Source: CAD feature listing. Evaluate the final solid. Frame: model axes, mm. A direction names the side the tool comes from. Round coordinates to 2 decimals unless told otherwise and drop trailing zeros. Loops run counter-clockwise (first coordinate to the right, second up) from the corner with the lowest first, then second, coordinate; pieces in that order, holes last. Notation, with made-up numbers: (21.25, 25) - (75.25, 25) arc R23 ccw to (75.25, 43) - close; hole circle Ø9 at (-23, 62.5). An arc over 180 degrees is marked (long way). One line per question, with ' | ' between items.
from build123d import *

# Parameters (mm, degrees)
SKETCH2_R           = 13.5
BOSS_EXTRUDE1_DEPTH = 8
SKETCH3_W           = 30
SKETCH3_H           = 34.126910457
BOSS_EXTRUDE2_DEPTH = 8
FILLET1_R           = 1


with BuildPart() as part:
    # Sketch2 → Boss-Extrude1 (new body)
    with BuildSketch(Plane.XY):
        with BuildLine():
            Line((22.912878475, 16.112283523), (-0.087121525, 16.112283523))
            Line((-0.087121525, 16.112283523), (-0.087121525, -17.887716477))
            Line((-0.087121525, -17.887716477), (22.912878475, -17.887716477))
            ThreePointArc((22.912878475, -17.887716477), (39.912878475, -0.887716477), (22.912878475, 16.112283523))
        make_face()
        with Locations((22.912878475, -0.887716477)):
            Circle(SKETCH2_R, mode=Mode.SUBTRACT)
    extrude(amount=BOSS_EXTRUDE1_DEPTH)

    # Sketch3 → Boss-Extrude2 (add)
    with BuildSketch(Plane.ZY.offset(0.087121525)):
        with Locations((4, -0.824261249)):
            Rectangle(SKETCH3_W, SKETCH3_H)
    extrude(amount=-BOSS_EXTRUDE2_DEPTH)

    # Fillet1
    fillet1_edges = [part.edges().sort_by_distance(p)[0] for p in [
        (7.912878475, -0.887716477, 8),
        (7.912878475, -0.887716477, 0),
    ]]
    fillet(fillet1_edges, radius=FILLET1_R)


solid = part.part
1. Section query B-B, the plane z = 6.5. Return loops of the section in (x, y), plus the area to 3 significant figures.
Worked out:
outline: (-0.09, -17.89) - (22.91, -17.89) arc R17 ccw to (22.91, 16.11) - (7.91, 16.11) - (7.91, 16.24) - (-0.09, 16.24) - close; hole circle Ø27 at (22.91, -0.89) | area: 664 mm2
2. Contact query for flat-ended pins moving along their axis: P1, Ø5, axis at x = 33.5, y = 10.5, coming from the +Z side; P2, Ø5, axis at x = 19.5, z = 2.5, coming from the +Y side; P3, Ø8, axis at y = -11.5, z = -0.5, coming from the +X side; P4, Ø6, axis at x = 19, z = -5.5, coming from the -Y side. Output: stop coordinate, or through.
Worked out:
P1: stops at z = 8 | P2: stops at y = 16.11 | P3: stops at x = 38.56 | P4: passes through
3. Section query D-D, the plane x = 32. Return loops of the section in (y, z).
Worked out:
outline: (-15.26, 0) - (-10.87, 0) - (-10.87, 8) - (-15.26, 8) - close; (9.1, 0) - (13.48, 0) - (13.48, 8) - (9.1, 8) - close
4. Section query C-C, the plane y = 9.5. Return loops of the section in (x, z), plus the area to 3 significant figures.
Worked out:
outline: (-0.09, -11) - (7.91, -11) - (7.91, -1) arc R1 cw to (8.91, 0) - (14.29, 0) - (14.29, 8) - (8.91, 8) arc R1 cw to (7.91, 9) - (7.91, 19) - (-0.09, 19) - close; (31.54, 0) - (36.37, 0) - (36.37, 8) - (31.54, 8) - close | area: 330 mm2
5. Access query for faces 1 (the flat face through (35, -8, 0)), 2 (the flat face through (35, -8, 8)), 3 (the flat face through (-0.087, -1, 4)). Directions: +Z, -Z, +X, -X, +Y, -Y. A direction counts if a zero-diameter tool reaches every point of the face in a straight line with its end or side. Return the directions, or none.
Worked out:
face 1: -Z, +X, +Y, -Y | face 2: +Z, +X, +Y, -Y | face 3: +Z, -Z, -X, +Y, -Y
6. Mould query, pull axis X, two halves, no side actions, for faces 4 (the flat face through (7.913, -1, -3)), 5 (the cylindrical face through (9.426, -0.294, 3.944)), 6 (the flat face through (16, 16.112, 4)). Classes: released by +X, released by -X, zero draft, split by the parting line, or undercut.
Worked out:
face 4: released by +X | face 5: undercut | face 6: zero draft
7. Material intervals for probe 1 along X at (y, z) = (-9.5, -9.5); probe 2 along Z at (x, y) = (11, 12.5); probe 3 along X at (y, z) = (2.5, 4.25), sorted ascending.
Worked out:
probe 1: x = -0.09 to 7.91 | probe 2: z = 0 to 8 | probe 3: x = -0.09 to 9.84, 35.98 to 39.57
8. Section query A-A, the plane x = 16.5. Return loops of the section in (y, z), plus the area to 3 significant figures.
Worked out:
outline: (-17.89, 0) - (-12.77, 0) - (-12.77, 8) - (-17.89, 8) - close; (10.99, 0) - (16.11, 0) - (16.11, 8) - (10.99, 8) - close | area: 81.9 mm2
